Input: part model. Units: mm. Frame: model coordinates. Face numbers are marked on the shaded views. A direction names the side the tool comes from. Round coordinates to 2 decimals unless told otherwise and drop trailing zeros. Loops run counter-clockwise (first coordinate to the right, second up) from the corner with the lowest first, then second, coordinate; pieces in that order, holes last.
(1) Line query: line 1 (Z direction, x = 3.75, y = 2.5); line 2 (Y direction, x = 1.85, z = 7.5); line 3 (Z direction, x = 2.35, y = 2.5). Output: solid intervals per line, ascending.
(2) Cut plane A-A, the plane z = 19. Output: boundary loops of the cut face in (x, y), and give its area (3 significant figures).
(3) First-contact query: pin 1 Ø9.5 at (y, z) = (5.5, 9) entering from -X; pin 2 Ø6 at (y, z) = (2.5, 7.5) entering from +X; pin 3 Ø1.6 at (x, z) = (6, 20) entering from +Y; pin 4 Ø4.5 at (y, z) = (2.5, 7.5) entering from -X. Flat tips, straight axial feed; report the tip coordinate or a pass-through.
(4) Access query for the marked faces 1, 2 and 3. Directions: +Z, -Z, +X, -X, +Y, -Y. A direction counts if a zero-diameter tool reaches every point of the face in a straight line with its end or side. Return the directions, or none.
(5) Cut plane B-B, the plane y = -9.5. Output: boundary loops of the cut face in (x, z), and give its area (3 significant figures).
(6) Cut plane C-C, the plane y = -5.25. Output: boundary loops of the cut face in (x, z), and give its area (3 significant figures).
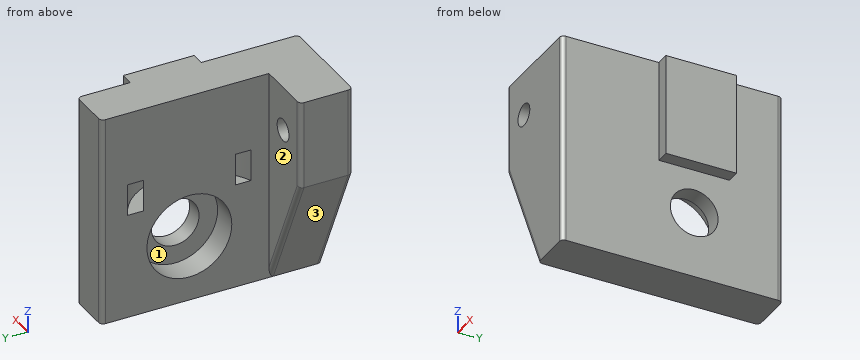
from build123d import *

# Parameters (mm, degrees)
BOSS_EXTRUDE1_DEPTH = 24
CUT_EXTRUDE1_REACH  = 37.26
SKETCH2_R           = 1.25
SKETCH2_W           = 1.5
SKETCH2_H           = 12.5
SKETCH3_R           = 2.7
CUT_EXTRUDE2_DEPTH  = 28.8298401
SKETCH4_R           = 4.8
CUT_EXTRUDE3_DEPTH  = 3
FILLET1_R           = 0.5
CUT_EXTRUDE4_DEPTH  = 3.6


with BuildPart() as part:
    # Sketch1 → Boss-Extrude1 (new body)
    with BuildSketch(Plane.XY):
        Polygon((5, 12.5), (0, 12.5), (0, -6.5), (-6.5, -6.5), (-6.5, -12.5), (5, -12.5), (5, -1.5), (6.5, -1.5), (6.5, 6.5), (5, 6.5), align=None)
    extrude(amount=BOSS_EXTRUDE1_DEPTH)

    # Sketch2 → Cut-Extrude1 (cut, up to next)
    with BuildSketch(Plane.XZ.offset(12.5), mode=Mode.PRIVATE) as cut_extrude1_sk1:
        with Locations((-3, 19)):
            Circle(SKETCH2_R)
    cut_extrude1_tool1 = extrude(cut_extrude1_sk1.sketch, amount=-CUT_EXTRUDE1_REACH, mode=Mode.PRIVATE) & part.part
    # Sketch2 → Cut-Extrude1 (cut, up to next)
    with BuildSketch(Plane.XZ.offset(12.5), mode=Mode.PRIVATE) as cut_extrude1_sk2:
        with Locations((5.75, 6.25)):
            Rectangle(SKETCH2_W, SKETCH2_H)
    cut_extrude1_tool2 = extrude(cut_extrude1_sk2.sketch, amount=-CUT_EXTRUDE1_REACH, mode=Mode.PRIVATE) & part.part
    # Sketch2 → Cut-Extrude1 (cut, up to next)
    with BuildSketch(Plane.XZ.offset(12.5), mode=Mode.PRIVATE) as cut_extrude1_sk3:
        Polygon((0, 0), (-6.5, 14), (-6.5, 0), align=None)
    cut_extrude1_tool3 = extrude(cut_extrude1_sk3.sketch, amount=-CUT_EXTRUDE1_REACH, mode=Mode.PRIVATE) & part.part
    add(cut_extrude1_tool1.solids().sort_by_distance((-3, -12.5, 19))[0], mode=Mode.SUBTRACT)
    add(cut_extrude1_tool2.solids().sort_by_distance((5.75, -12.5, 6.25))[0], mode=Mode.SUBTRACT)
    add(cut_extrude1_tool3.solids().sort_by_distance((-4.333333, -12.5, 4.666667))[0], mode=Mode.SUBTRACT)

    # Sketch3 → Cut-Extrude2 (cut, through all)
    with BuildSketch(Plane.ZY):
        with Locations(Location((7.5, 2.5, 0), (0, 0, 270))):
            Circle(SKETCH3_R)
    extrude(amount=-CUT_EXTRUDE2_DEPTH, mode=Mode.SUBTRACT)

    # Sketch4 → Cut-Extrude3 (cut)
    with BuildSketch(Plane.ZY):
        with Locations(Location((7.5, 2.5, 0), (0, 0, 270))):
            Circle(SKETCH4_R)
    extrude(amount=-CUT_EXTRUDE3_DEPTH, mode=Mode.SUBTRACT)

    # Fillet1
    fillet1_edges = [part.edges().sort_by_distance(p)[0] for p in [
        (5, -12.5, 12),
        (-6.5, -12.5, 19),
        (-6.5, -6.5, 19),
        (0, 12.5, 12),
        (5, 12.5, 12),
        (-3.25, -12.5, 7),
        (-3.25, -6.5, 7),
    ]]
    fillet(fillet1_edges, radius=FILLET1_R)

    # Sketch6 → Cut-Extrude4 (cut)
    with BuildSketch(Plane(origin=(0, 0, 12), x_dir=(-1, 0, 0), z_dir=(0, 0, -1))):
        with BuildLine():
            Line((0, 7.69614), (0, 9.48283))
            ThreePointArc((0, 9.48283), (-4.6, 2.5), (0, -4.48283))
            Line((0, -4.48283), (0, -2.69614))
            ThreePointArc((0, -2.69614), (-2.999993872, 2.5), (0, 7.69614))
        make_face()
    extrude(amount=-CUT_EXTRUDE4_DEPTH, mode=Mode.SUBTRACT)


solid = part.part
Reported:
1. line 1: z = 0 to 4.8, 10.2 to 12, 15.6 to 24
1. line 2: y = -12.5 to -2.3, 7.3 to 12.5
1. line 3: z = 0 to 2.7, 12.3 to 24
2. outline: (-6.5, -12) arc R0.5 ccw to (-6, -12.5) - (-4.25, -12.5) - (-4.25, -6.5) - (-6, -6.5) arc R0.5 ccw to (-6.5, -7) - close; (-1.75, -12.5) - (4.5, -12.5) arc R0.5 ccw to (5, -12) - (5, -1.5) - (6.5, -1.5) - (6.5, 6.5) - (5, 6.5) - (5, 12) arc R0.5 ccw to (4.5, 12.5) - (0.5, 12.5) arc R0.5 ccw to (0, 12) - (0, -6.5) - (-1.75, -6.5) - close
2. area: 161 mm2
3. pin 1: stops at x = 0
3. pin 2: stops at x = 5
3. pin 3: stops at y = 6.5
3. pin 4: passes through
4. face 1: -X
4. face 2: +Z, -Z, -X, +Y
4. face 3: -Z, -X, +Y, -Y
5. outline: (-6.5, 14) - (0, 0) - (5, 0) - (5, 24) - (-6.5, 24) - close; hole circle Ø2.5 at (-3, 19)
5. area: 226 mm2
6. outline: (0, 0) - (5, 0) - (5, 24) - (0, 24) - close
6. area: 120 mm2
